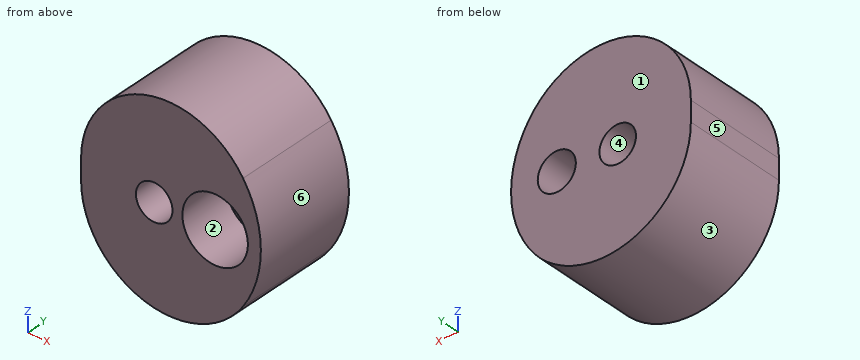
from build123d import *

# Parameters (mm, degrees)
SKETCH1_R           = 1.2
SKETCH1_R_2         = 1.25
BOSS_EXTRUDE1_DEPTH = 7
SKETCH3_R           = 2.15
CUT_EXTRUDE3_DEPTH  = 3.5
FILLET1_R           = 5.8


with BuildPart() as part:
    # Sketch1 → Boss-Extrude1 (new body)
    with BuildSketch(Plane(origin=(0, 0, 0), x_dir=(1, 0, 0), z_dir=(0, 1, 0))):
        with BuildLine():
            Line((9.45, 19.218429014), (9.45, 9.028237652))
            ThreePointArc((9.45, 9.028237652), (21.25, 14.123333333), (9.45, 19.218429014))
        make_face()
        with Locations((14.25, 14.123333333)):
            Circle(SKETCH1_R, mode=Mode.SUBTRACT)
        with Locations((18.25, 14.123333333)):
            Circle(SKETCH1_R_2, mode=Mode.SUBTRACT)
    extrude(amount=BOSS_EXTRUDE1_DEPTH)

    # Sketch3 → Cut-Extrude3 (cut)
    with BuildSketch(Plane.XZ):
        with Locations((18.25, -14.123333333)):
            Circle(SKETCH3_R)
    extrude(amount=-CUT_EXTRUDE3_DEPTH, mode=Mode.SUBTRACT)

    # Fillet1
    fillet1_edges = [part.edges().sort_by_distance(p)[0] for p in [
        (9.45, 3.5, -9.028237652),
        (9.45, 3.5, -19.218429014),
    ]]
    fillet(fillet1_edges, radius=FILLET1_R)


solid = part.part
Part model, mm, in its own coordinate system. Face numbers are marked on the shaded views. A direction names the side the tool comes from. Coordinates: 2 decimals unless noted, no trailing zeros. Order: outer loops, then holes, each group sorted by start corner. A loop starts at its lowest first (then second) coordinate and runs counter-clockwise, first axis right, second up.
(1) Pin check, flat tips, straight feed: pin 1 Ø1 at (x, y) = (13.5, 5) entering from +Z; pin 2 Ø1.5 at (x, z) = (18.25, -14.12) entering from -Y. Stop position of each tip, or through.
Check sheet entries:
pin 1: stops at z = -7.8
pin 2: passes through
(2) Tool access for the marked faces 1 and 2: list every direction of +Z, -Z, +X, -X, +Y, -Y with a clear straight run to the whole face (end or side of a thin tool).
Check sheet entries:
face 1: +Z, -Z, +X, -X, +Y
face 2: -Y
(3) Pull direction X, two halves, no side cores. Call the marked faces 3, 4, 5 and 6: pulls with the +X half, pulls with the -X half, needs draft (parallel to the pull), parting line crosses it, or undercut.
Check sheet entries:
face 3: parting line crosses it
face 4: undercut
face 5: pulls with the -X half
face 6: pulls with the +X half
(4) Slice it at B-B, the plane y = 2.25. Write the cut outline in (x, z).
Check sheet entries:
outline: (9.45, -14.79) arc R5.8 ccw to (20.08, -17.99) arc R7 ccw to (20.08, -10.25) arc R5.8 ccw to (9.45, -13.46) - close; hole circle Ø2.4 at (14.25, -14.12); hole circle Ø4.3 at (18.25, -14.12)
(5) Slice it at C-C, the plane x = 18.25. Write the cut outline in (y, z), and give its area (3 significant figures).
Check sheet entries:
outline: (0, -19.75) - (7, -19.75) - (7, -15.37) - (3.5, -15.37) - (3.5, -16.27) - (0, -16.27) - close; (0, -11.97) - (3.5, -11.97) - (3.5, -12.87) - (7, -12.87) - (7, -8.5) - (0, -8.5) - close
area: 55.0 mm2
(6) Slice it at A-A, the plane x = 14.25. Write the cut outline in (y, z), and give its area (3 significant figures).
Check sheet entries:
outline: (0, -20.5) - (7, -20.5) - (7, -15.32) - (0, -15.32) - close; (0, -12.92) - (7, -12.92) - (7, -7.75) - (0, -7.75) - close
area: 72.5 mm2
(7) Slice it at D-D, the plane z = -17. Write the cut outline in (x, y), and give its area (3 significant figures).
Check sheet entries:
outline: (9.89, 0) - (20.63, 0) - (20.63, 7) - (9.89, 7) - close
area: 75.2 mm2
(8) Probe L1, parallel to X at y = 2, z = -14; L2, parallel to Z at x = 13.5, y = 4; L3, parallel to Z at x = 14.25, y = 4.75. List the from-to ranges inside material, lowest first.
Check sheet entries:
L1: x = 9.45 to 13.06, 15.44 to 16.1, 20.4 to 21.25
L2: z = -20.32 to -15.06, -13.19 to -7.93
L3: z = -20.5 to -15.32, -12.92 to -7.75
